```python
from build123d import *

# Parameters (mm, degrees)
BOSS_EXTRUDE1_DEPTH = 50
FILLET1_R           = 10
FILLET2_R           = 5
BOSS_EXTRUDE3_DEPTH = 2
BOSS_EXTRUDE4_DEPTH = 2


with BuildPart() as part:
    # Sketch2 → Boss-Extrude1 (new, symmetric)
    with BuildSketch(Plane.XY.offset(-83)):
        with BuildLine():
            Line((-4, 165.635164807), (-4, 147))
            Line((-4, 147), (-9, 147))
            Line((-9, 147), (-9, 165.635164807))
            ThreePointArc((-9, 165.635164807), (-8.747881204, 168.373777595), (-8, 171.020329614))
            ThreePointArc((-8, 171.020329614), (-1.677925359, 180.988070116), (8, 187.74545417))
            ThreePointArc((8, 187.74545417), (10.183300133, 189.589417077), (11, 192.328029865))
            Line((11, 192.328029865), (11, 253.25))
            Line((11, 253.25), (16, 253.25))
            Line((16, 253.25), (16, 192.328029865))
            ThreePointArc((16, 192.328029865), (14.366600265, 186.85080429), (10, 183.162878475))
            ThreePointArc((10, 183.162878475), (1.935062201, 177.531725097), (-3.333333333, 169.225274679))
            ThreePointArc((-3.333333333, 169.225274679), (-3.831920803, 167.460906665), (-4, 165.635164807))
        make_face()
    extrude(amount=BOSS_EXTRUDE1_DEPTH, both=True)

    # Fillet1
    fillet1_edges = [part.edges().sort_by_distance(p)[0] for p in [
        (13.5, 253.25, -133),
        (13.5, 253.25, -33),
    ]]
    fillet(fillet1_edges, radius=FILLET1_R)

    # Fillet2
    fillet2_edges = [part.edges().sort_by_distance(p)[0] for p in [
        (-6.5, 147, -133),
        (-6.5, 147, -33),
    ]]
    fillet(fillet2_edges, radius=FILLET2_R)

    # Sketch4 → Boss-Extrude3 (add, symmetric)
    with BuildSketch(Plane.XY.offset(-53)):
        with BuildLine():
            Line((10.095389312, 240.764602561), (-8.095389312, 190.78584905))
            ThreePointArc((-8.095389312, 190.78584905), (-8.772116295, 188.260269565), (-9, 185.6555469))
            Line((-9, 185.6555469), (-9, 165.635164807))
            ThreePointArc((-9, 165.635164807), (-8.747881204, 168.373777595), (-8, 171.020329614))
            ThreePointArc((-8, 171.020329614), (-1.677925359, 180.988070116), (8, 187.74545417))
            ThreePointArc((8, 187.74545417), (10.183300133, 189.589417077), (11, 192.328029865))
            Line((11, 192.328029865), (11, 245.894904711))
            ThreePointArc((11, 245.894904711), (10.772116295, 243.290182046), (10.095389312, 240.764602561))
        make_face()
    extrude(amount=BOSS_EXTRUDE3_DEPTH, both=True)

    # Sketch5 → Boss-Extrude4 (add, symmetric)
    with BuildSketch(Plane(origin=(0, 0, -113), x_dir=(-1, 0, 0), z_dir=(0, 0, -1))):
        with BuildLine():
            Line((-11, 245.894904711), (-11, 192.328029865))
            ThreePointArc((-11, 192.328029865), (-10.183300133, 189.589417077), (-8, 187.74545417))
            ThreePointArc((-8, 187.74545417), (1.677925359, 180.988070116), (8, 171.020329614))
            ThreePointArc((8, 171.020329614), (8.747881204, 168.373777595), (9, 165.635164807))
            Line((9, 165.635164807), (9, 185.6555469))
            ThreePointArc((9, 185.6555469), (8.772116295, 188.260269565), (8.095389312, 190.78584905))
            Line((8.095389312, 190.78584905), (-10.095389312, 240.764602561))
            ThreePointArc((-10.095389312, 240.764602561), (-10.772116295, 243.290182046), (-11, 245.894904711))
        make_face()
    extrude(amount=BOSS_EXTRUDE4_DEPTH, both=True)


solid = part.part
```
Check sheet for the modelled part. Datum: model origin and axes. Units: mm. A direction names the side the tool comes from. Give positions to 0.01 mm unless a question says otherwise; leave off trailing zeros. Write each loop counter-clockwise with the first axis right and the second up, starting at its lowest first coordinate (ties: lowest second). Pieces come first, ordered by that corner, then holes. Notation, with made-up numbers: (75, -6) -> (90, -6) arc R29 ccw to (90, 17) -> close; hole circle Ø10 at (80.25, 83.5). An arc over 180 degrees is marked (long way). Use CSV: the item, a comma, the result in double quotes. Start each with the question number.
Q1. Release check for a two-part mould opening along Z. For faces 4 (the cylindrical face through (10.161, 189.556, -82.608)), 5 (the cylindrical face through (-7, 148, -131)), 6 (the cylindrical face through (-8.766, 188.296, -52.972)) record: +Z half, -Z half, draft (parallel to the pull), parting line (faces both ways), or undercut.
Q2. Tool access check on faces 1 (the cylindrical face through (10.161, 189.556, -123.874)), 2 (the cylindrical face through (2, 177.6, -82.3)), 3 (the cylindrical face through (-1.79, 180.87, -41.87)). Record the directions out of +Z, -Z, +X, -X, +Y, -Y that give a thin tool (end or side, any length) a straight path to the whole face; none if there is none.
Q3. Cross-section at A-A on z = -65.5. Enter the section's corners in (x, y), and give its area (3 significant figures).
Q4. Depth check by flat-ended pin: P1, Ø6, axis at x = 0, y = 190.5, coming from the +Z side; P2, Ø18.5, axis at y = 234, z = -100.5, coming from the -X side; P3, Ø10, axis at y = 165.5, z = -90, coming from the +X side. Enter the tip coordinate at first touch or a pass-through.
Q5. Scan lines: line 1 along Z through (x, y) = (-7, 175.5); line 2 along X through (y, z) = (215.5, -48); line 3 along X through (y, z) = (160, -125). Record each from-to range of solid material in increasing order.
Q6. Cross-section at D-D on x = -6.5. Enter the section's corners in (y, z).
Q7. Cross-section at B-B on x = 1. Enter the section's corners in (y, z), and give its area (3 significant figures).
Q8. Cross-section at C-C on y = 159.5. Enter the section's corners in (x, z).
Working result:
1,face 4,"undercut"
1,face 5,"-Z half"
1,face 6,"draft"
2,face 1,"-Z, -X, +Y"
2,face 2,"+Z, -Z, +X, -Y"
2,face 3,"+Z, -X, +Y"
3,outline,"(-9, 147) -> (-4, 147) -> (-4, 165.64) arc R10 cw to (-3.33, 169.23) arc R25 cw to (10, 183.16) arc R10 ccw to (16, 192.33) -> (16, 253.25) -> (11, 253.25) -> (11, 192.33) arc R5 cw to (8, 187.75) arc R30 ccw to (-8, 171.02) arc R15 ccw to (-9, 165.64) -> close"
3,area,"573 mm^2"
4,P1,"stops at z = -51"
4,P2,"stops at x = 11"
4,P3,"stops at x = -2.8"
5,line 1,"z = -115 to -111, -55 to -51"
5,line 2,"x = 11 to 16"
5,line 3,"x = -9 to -4"
6,outline,"(147, -128) arc R5 ccw to (152, -133) -> (174.31, -133) -> (174.31, -115) -> (195.17, -115) -> (195.17, -111) -> (174.31, -111) -> (174.31, -55) -> (195.17, -55) -> (195.17, -51) -> (174.31, -51) -> (174.31, -33) -> (152, -33) arc R5 ccw to (147, -38) -> close"
7,outline,"(176.5, -133) -> (183.47, -133) -> (183.47, -115) -> (215.78, -115) -> (215.78, -111) -> (183.47, -111) -> (183.47, -55) -> (215.78, -55) -> (215.78, -51) -> (183.47, -51) -> (183.47, -33) -> (176.5, -33) -> close"
7,area,"955 mm^2"
8,outline,"(-9, -133) -> (-4, -133) -> (-4, -33) -> (-9, -33) -> close"
